```python
from build123d import *

# Parameters (mm, degrees)
SKETCH1_W                      = 20
SKETCH1_H                      = 28
BOSS_EXTRUDE1_DEPTH            = 28
SKETCH2_W                      = 15
SKETCH2_H                      = 25.5
CUT_EXTRUDE1_DEPTH             = 25.5
CUT_EXTRUDE2_REACH             = 12
CUT_EXTRUDE2_DIRECTION_2_REACH = 12


with BuildPart() as part:
    # Sketch1 → Boss-Extrude1 (new body)
    with BuildSketch(Plane(origin=(0, 0, 0), x_dir=(1, 0, 0), z_dir=(0, 1, 0))):
        with Locations((10, -14)):
            Rectangle(SKETCH1_W, SKETCH1_H)
    extrude(amount=BOSS_EXTRUDE1_DEPTH)

    # Sketch2 → Cut-Extrude1 (cut)
    with BuildSketch(Plane(origin=(0, 28, 0), x_dir=(1, 0, 0), z_dir=(0, 1, 0))):
        with Locations((10, -15.25)):
            Rectangle(SKETCH2_W, SKETCH2_H)
    extrude(amount=-CUT_EXTRUDE1_DEPTH, mode=Mode.SUBTRACT)

    # Sketch3 → Cut-Extrude2 (cut, up to next)
    with BuildSketch(Plane.ZY.offset(-10), mode=Mode.PRIVATE) as cut_extrude2_sk1:
        Polygon((4, 28), (4, 25.5), (25.5, 4), (28, 4), (28, 28), align=None)
    cut_extrude2_tool1 = extrude(cut_extrude2_sk1.sketch, amount=-CUT_EXTRUDE2_REACH, mode=Mode.PRIVATE) & part.part
    add(cut_extrude2_tool1.solids().sort_by_distance((10, 19.239157, 19.239157))[0], mode=Mode.SUBTRACT)

    # Sketch3 → Cut-Extrude2 direction 2 (cut, up to next)
    with BuildSketch(Plane.ZY.offset(-10), mode=Mode.PRIVATE) as cut_extrude2_direction_2_sk1:
        Polygon((4, 28), (4, 25.5), (25.5, 4), (28, 4), (28, 28), align=None)
    cut_extrude2_direction_2_tool1 = extrude(cut_extrude2_direction_2_sk1.sketch, amount=CUT_EXTRUDE2_DIRECTION_2_REACH, mode=Mode.PRIVATE) & part.part
    add(cut_extrude2_direction_2_tool1.solids().sort_by_distance((10, 19.239157, 19.239157))[0], mode=Mode.SUBTRACT)


solid = part.part
```
Source: CAD feature listing. Evaluate the final solid. Frame: model axes, mm. A direction names the side the tool comes from. Coordinates: 2 decimals unless noted, no trailing zeros. Order: outer loops, then holes, each group sorted by start corner. A loop starts at its lowest first (then second) coordinate and runs counter-clockwise, first axis right, second up. Notation, with made-up numbers: M 14.5,-22 L 66.5,-22 A16 ccw 66.5,-1 Z; hole C 86.5,-27 d7. An arc over 180 degrees is marked long. Write each question's results on one line, items separated by ' | '. Start each with the question number.
1) Contact query for flat-ended pins moving along their axis: pin 1 Ø0.8 at (x, y) = (18.5, 26.5) entering from +Z; pin 2 Ø2 at (x, z) = (1, 27) entering from +Y; pin 3 Ø4.5 at (x, y) = (12.5, 21) entering from +Z. Output: stop coordinate, or through.
2) Section query A-A (y = 23.75). Return the cut outline in (x, z).
3) Section query C-C (x = 13.5). Return the cut outline in (y, z).
4) Section query D-D (x = 2). Return the cut outline in (y, z), plus the area to 3 significant figures.
5) Section query B-B (z = 3.5). Return the cut outline in (x, y), plus the area to 4 significant figures.
6) Draft query along X for faces 1 (the face through (0, 11, 11)), 2 (the face through (20, 11, 11)), 3 (the face through (1.3, 14.9, 14.6)), 4 (the face through (10, 15, 2.5)). Return one class per face: released by +X, released by -X, zero draft, split by the parting line, or undercut.
7) Line query: line 1 (X direction, y = 20.5, z = 6.5); line 2 (Z direction, x = 10.75, y = 5.75). Output: solid intervals per line, ascending. Write a range as from..to.
8) Access query for faces 5 (the face through (10, 14, 0)), 6 (the face through (2.5, 10, 10)), 7 (the face through (19, 4, 27)). Directions: +Z, -Z, +X, -X, +Y, -Y. A direction counts if a zero-diameter tool reaches every point of the face in a straight line with its end or side. Return the directions, or none.
Answers:
1) pin 1: stops at z = 4 | pin 2: stops at y = 4 | pin 3: stops at z = 2.5
2) outline: M 0,0 L 20,0 L 20,5.75 L 17.5,5.75 L 17.5,2.5 L 2.5,2.5 L 2.5,5.75 L 0,5.75 Z
3) outline: M 0,0 L 28,0 L 28,2.5 L 2.5,2.5 L 2.5,28 L 0,28 Z
4) outline: M 0,0 L 28,0 L 28,4 L 25.5,4 L 4,25.5 L 4,28 L 0,28 Z | area: 439 mm^2
5) outline: M 0,0 L 20,0 L 20,28 L 17.5,28 L 17.5,2.5 L 2.5,2.5 L 2.5,28 L 0,28 Z | area: 177.5 mm^2
6) face 1: released by -X | face 2: released by +X | face 3: zero draft | face 4: undercut
7) line 1: x = 0..2.5, 17.5..20 | line 2: z = 0..2.5
8) face 5: -Z, +X, -X, +Y, -Y | face 6: +Z, +Y | face 7: +Z, +X, -X, +Y
